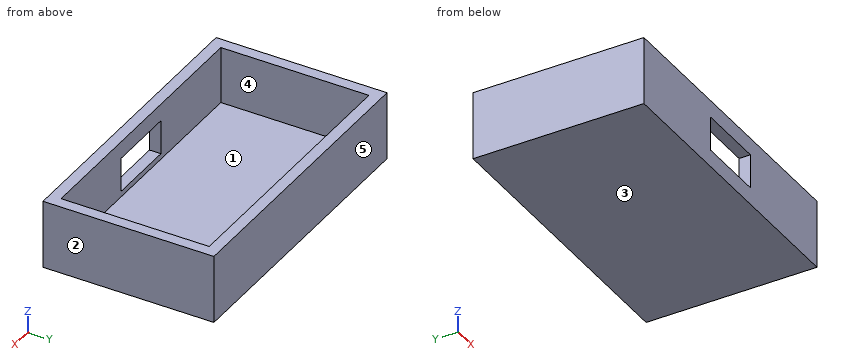
```python
from build123d import *

# Parameters (mm, degrees)
SKETCH1_W           = 130
SKETCH1_H           = 30
BOSS_EXTRUDE1_DEPTH = 75
SHELL1_T            = -5
CUT_EXTRUDE1_REACH  = 77
SKETCH2_W           = 30
SKETCH2_H           = 15


with BuildPart() as part:
    # Sketch1 → Boss-Extrude1 (new body)
    with BuildSketch(Plane(origin=(0, 0, 0), x_dir=(1, 0, 0), z_dir=(0, 1, 0))):
        with Locations((65, 15)):
            Rectangle(SKETCH1_W, SKETCH1_H)
    extrude(amount=BOSS_EXTRUDE1_DEPTH)

    # Shell1
    shell1_openings = [part.faces().sort_by_distance(p)[0] for p in [
        (65, 37.5, 0),
    ]]
    offset(amount=SHELL1_T, openings=shell1_openings, kind=Kind.INTERSECTION)

    # Sketch2 → Cut-Extrude1 (cut, up to next)
    with BuildSketch(Plane.XZ, mode=Mode.PRIVATE) as cut_extrude1_sk1:
        with Locations((65, -15)):
            Rectangle(SKETCH2_W, SKETCH2_H)
    cut_extrude1_tool1 = extrude(cut_extrude1_sk1.sketch, amount=-CUT_EXTRUDE1_REACH, mode=Mode.PRIVATE) & part.part
    add(cut_extrude1_tool1.solids().sort_by_distance((65, 0, -15))[0], mode=Mode.SUBTRACT)


solid = part.part
```
Can you work these out from the model? Positions are in its coordinate system, mm. Face numbers are marked on the shaded views. A direction names the side the tool comes from. Coordinates: 2 decimals unless noted, no trailing zeros. Loops run counter-clockwise (first coordinate to the right, second up) from the corner with the lowest first, then second, coordinate; pieces in that order, holes last.
1) For pin 1 (1.5 mm diameter, centred on x = 69.5, z = -15.5, fed in from -Y); pin 2 (19.5 mm diameter, centred on x = 48.5, y = 42, fed in from +Z), each with a flat end and sliding along its axis, tell me the tip position at first contact or that it passes through.
2) Imagine slicing it at A-A on z = -5.75. List the corners of the cut face in (x, y) for me.
3) I need wall thicknesses on probe 1 along Y at (x, z) = (107.5, -22.25); probe 2 along X at (y, z) = (51, -22.25); probe 3 along Z at (x, y) = (65, 3). Which ranges of each line are inside material? Lowest first, please.
4) Thinking about a two-plate mould opening in Y: for the marked faces 3, 4 and 5, which applies, pulls with the +Y half, pulls with the -Y half, needs draft (parallel to the pull), parting line crosses it, or undercut?
5) Imagine slicing it at D-D on z = -13.75. List the corners of the cut face in (x, y) for me.
6) Imagine slicing it at C-C on y = 53.5. List the corners of the cut face in (x, z) for me.
7) Which directions (+Z, -Z, +X, -X, +Y, -Y) give clear straight access to the entire face, cutting with the end or side of a thin tool? Please do the marked faces 1 and 2.
8) Imagine slicing it at B-B on x = 76. List the corners of the cut face in (y, z) for me, plus the area to 3 significant figures.
Completed:
1. pin 1: stops at y = 70
1. pin 2: stops at z = -25
2. outline: (0, 0) - (130, 0) - (130, 75) - (0, 75) - close; hole (5, 5) - (125, 5) - (125, 70) - (5, 70) - close
3. probe 1: y = 0 to 5, 70 to 75
3. probe 2: x = 0 to 5, 125 to 130
3. probe 3: z = -30 to -22.5, -7.5 to 0
4. face 3: needs draft
4. face 4: undercut
4. face 5: pulls with the +Y half
5. outline: (0, 0) - (50, 0) - (50, 5) - (5, 5) - (5, 70) - (125, 70) - (125, 5) - (80, 5) - (80, 0) - (130, 0) - (130, 75) - (0, 75) - close
6. outline: (0, -30) - (130, -30) - (130, 0) - (125, 0) - (125, -25) - (5, -25) - (5, 0) - (0, 0) - close
7. face 1: +Z
7. face 2: +Z, -Z, +X, +Y, -Y
8. outline: (0, -30) - (75, -30) - (75, 0) - (70, 0) - (70, -25) - (5, -25) - (5, -22.5) - (0, -22.5) - close; (0, -7.5) - (5, -7.5) - (5, 0) - (0, 0) - close
8. area: 550 mm2
